from build123d import *

# Parameters (mm, degrees)
BOSS_EXTRUDE12_DEPTH = 60
BOSS_EXTRUDE13_DEPTH = 8
SKETCH3_W            = 20
SKETCH3_H            = 60
CUT_EXTRUDE1_DEPTH   = 10


with BuildPart() as part:
    # Sketch1 → Boss-Extrude12 (new body)
    with BuildSketch(Plane(origin=(0, 0, 0), x_dir=(1, 0, 0), z_dir=(0, 1, 0))):
        with BuildLine():
            Line((3, 47), (3, 30))
            Line((3, 30), (0, 30))
            Line((0, 30), (0, 0))
            Line((0, 0), (-2, 0))
            Line((-2, 0), (-2, 32))
            Line((-2, 32), (1, 32))
            Line((1, 32), (1, 45))
            Line((1, 45), (0.176102142, 45))
            add(Edge.make_bspline(
                [(-18.386432119, 28), (-18.281589374, 28.071011485), (-18.076006872, 28.210643772), (-17.632017964, 28.509033814), (-16.788752159, 29.127765228), (-15.266101597, 30.436706514), (-13.281769764, 32.578807621), (-11.116323446, 35.322397153), (-8.327983452, 38.971629637), (-4.796332276, 42.989291988), (-1.605396872, 44.667429051), (0.176102142, 45)],
                knots=[0.007315744, 0.007315744, 0.007315744, 0.007315744, 0.023228008, 0.039140272, 0.0709648, 0.134613856, 0.261911967, 0.389210078, 0.516508189, 0.771104411, 1.025700634, 1.025700634, 1.025700634, 1.025700634], degree=3))
            Line((-18.386432119, 28), (-34.105031298, 28))
            Line((-34.105031298, 28), (-45, 45.32952773))
            Line((-45, 45.32952773), (-45, 0))
            Line((-45, 0), (-47, 0))
            Line((-47, 0), (-47, 52.268387809))
            Line((-47, 52.268387809), (-33, 30))
            Line((-33, 30), (-19, 30))
            add(Edge.make_bspline(
                [(0, 47), (-8.735842334, 45.522262704), (-12.411198706, 34.462689008), (-19, 30)],
                knots=[0, 0, 0, 0, 1, 1, 1, 1], degree=3))
            Line((0, 47), (3, 47))
        make_face()
    extrude(amount=BOSS_EXTRUDE12_DEPTH)

    # Sketch2 → Boss-Extrude13 (add)
    with BuildSketch(Plane(origin=(0, 0, -30), x_dir=(-1, 0, 0), z_dir=(0, 0, -1))):
        with BuildLine():
            Line((33, 0), (19, 0))
            Line((19, 0), (19, 2.423963318))
            ThreePointArc((19, 2.423963318), (26, 2), (33, 2.423963318))
            Line((33, 2.423963318), (33, 0))
        make_face()
    extrude(amount=BOSS_EXTRUDE13_DEPTH)

    # Sketch3 → Cut-Extrude1 (cut)
    with BuildSketch(Plane(origin=(0, 0, 0), x_dir=(0, 0, -1), z_dir=(1, 0, 0))):
        with Locations((10, 30)):
            Rectangle(SKETCH3_W, SKETCH3_H)
    extrude(amount=-CUT_EXTRUDE1_DEPTH, mode=Mode.SUBTRACT)


solid = part.part
Design review of the part built by this model. Coordinates are the model's own, in mm. A direction names the side the tool comes from. Coordinates: 2 decimals unless noted, no trailing zeros. Loops run counter-clockwise (first coordinate to the right, second up) from the corner with the lowest first, then second, coordinate; pieces in that order, holes last. Notation, with made-up numbers: M -39.5,7 L -32.5,7 A30 ccw -32.5,36 Z; hole C 76.25,79 d6. An arc over 180 degrees is marked long. Answer as CSV lines item,"result".
Item 1: Add section C-C on x = -29.5. State the section outline as (y, z) points.
Answer list:
outline,"M 0,-38 L 2.11,-38 L 2.11,-30 L 60,-30 L 60,-28 L 0,-28 Z"
Item 2: Add section D-D on z = -14. State the section outline as (x, y) points.
Answer list:
outline,"M -47,0 L -45,0 L -45,60 L -47,60 Z"
Item 3: For probe 1 along X at (y, z) = (33, -25); probe 2 along X at (y, z) = (31.5, -35); probe 3 along Z at (x, y) = (-22.5, 36), list the stretches that pass through material, from the lowest coordinate up.
Answer list:
probe 1,"-47 to -45, -2 to 0"
probe 2,"-47 to -45, -38.51 to -36.14, -13.93 to -11.38, 1 to 3"
probe 3,"-30 to -28"
Item 4: Add section B-B on z = -36.5. Count the separate pieces of the cut face and the enclosed holes in it, plus the area to 3 significant figures.
Answer list:
separate pieces,"5"
enclosed holes,"0"
area,"563 mm²"
Item 5: For P1, Ø6, axis at x = -33, z = -43, coming from the -Y side; P2, Ø11, axis at y = 17.5, z = -23, coming from the +X side; P3, Ø3.5, axis at x = 2, y = 20.5, coming from the +Z side; P4, Ø4, axis at x = -26.5, y = 27.5, coming from the -Z side, all flat-tipped, find the tip position at first contact; note any pin that passes through.
Answer list:
P1,"through"
P2,"x = 0"
P3,"z = -30"
P4,"z = -30"
Item 6: The part is to be moulded in two halves that separate along X. For faces 4 (the face through (-1, 30, -32)), 5 (the face through (-26, 1, -38)), 6 (the face through (1, 30, -47)), 7 (the face through (0, 30, -25)), say which applies: pulls with the +X half, pulls with the -X half, needs draft (parallel to the pull), parting line crosses it, or undercut.
Answer list:
face 4,"undercut"
face 5,"undercut"
face 6,"needs draft"
face 7,"pulls with the +X half"
Item 7: Machinability: for faces 1 (the face through (-39.476, 29.58, -36.543)), 2 (the face through (2, 30, -30)), 3 (the face through (-26, 2, -34)), which of the approach directions +Z, -Z, +X, -X, +Y, -Y give a long, thin tool a straight path to every point of the face, cutting with its end or side? Answer none if there is none.
Answer list:
face 1,"+Z, +Y, -Y"
face 2,"+Z, +X, +Y, -Y"
face 3,"-Z, +Y"
Item 8: Add section A-A on z = -22.5. State the section outline as (x, y) points, plus the area to 3 significant figures.
Answer list:
outline,"M -47,0 L -45,0 L -45,60 L -47,60 Z; M -2,0 L 0,0 L 0,60 L -2,60 Z"
area,"240 mm²"
